Here's how the part is built. I have some questions about the finished solid (model axes, mm). A direction names the side the tool comes from. Give positions to 0.01 mm unless a question says otherwise; leave off trailing zeros. Loops run counter-clockwise (first coordinate to the right, second up) from the corner with the lowest first, then second, coordinate; pieces in that order, holes last. Notation, with made-up numbers: (45.5, 33.5) -> (49.5, 33.5) arc R27 ccw to (49.5, 52.5) -> close; hole circle Ø8 at (-22.75, 47.25). An arc over 180 degrees is marked (long way). Answer in a Markdown table with one row per item. Add a question column.
Item 1: If we section it at B-B (z = 14.5): Write out the boundary of the cut face in (x, y).
Item 2: If I drill on line 1 (Y direction, x = 10, z = 10); line 2 (Y direction, x = 18.85, z = 47); line 3 (Y direction, x = 7.25, z = 5.5), over which ranges is the centre line in solid material (lowest first)?
Item 3: Which directions (+Z, -Z, +X, -X, +Y, -Y) give clear straight access to the entire face, cutting with the end or side of a thin tool? Please do faces 1 (the face through (11.77, 16.62, -2.99)), 2 (the face through (10, 4.8, -2)), 3 (the face through (9, 32.3, 32)).
Item 4: We'd pull the mould along Z, two halves only. Please class faces 4 (the face through (9, 25, 61)), 5 (the face through (9, 9, 50.5)), 6 (the face through (10.14, 48.64, -2.43)), 7 (the face through (5.326, 36.472, -0.986)): released by +Z, released by -Z, zero draft, split by the parting line, or undercut.
Item 5: For P1, Ø1.2, axis at x = 13.5, z = -1.5, coming from the -Y side; P2, Ø1.2, axis at x = 8.5, y = 10.5, coming from the -Z side; P3, Ø1.5, axis at x = 10, y = 35.5, coming from the -Z side, each with a flat end and sliding along its axis, tell me the tip position at first contact or that it passes through.
Item 6: If we section it at A-A (z = 47): Write out the boundary of the cut face in (x, y).
Item 7: If we section it at D-D (z = 55): Write out the boundary of the cut face in (x, y), then the cut area to 3 significant figures.
Item 8: If we section it at C-C (y = 6): Write out the boundary of the cut face in (x, z).
```python
from build123d import *

# Parameters (mm, degrees)
SKETCH1_W           = 20
SKETCH1_H           = 50
BOSS_EXTRUDE1_DEPTH = 66
SKETCH2_R           = 4.9
BOSS_EXTRUDE2_DEPTH = 2
SKETCH3_R           = 2.4
BOSS_EXTRUDE3_DEPTH = 2
SKETCH4_R           = 1.5
CUT_EXTRUDE1_DEPTH  = 20
CUT_EXTRUDE2_START  = -18
CUT_EXTRUDE2_DEPTH  = 18
CUT_EXTRUDE3_REACH  = 86.735
SKETCH8_W           = 20
SKETCH8_H           = 4.8
BOSS_EXTRUDE4_DEPTH = 4
FILLET1_R           = 5


# Read off the part's stored shape, not the designer's step: Cut-Extrude2
with BuildPart() as part:
    # Sketch1 → Boss-Extrude1 (new body)
    with BuildSketch(Plane.XY):
        with Locations((10, 25)):
            Rectangle(SKETCH1_W, SKETCH1_H)
    extrude(amount=BOSS_EXTRUDE1_DEPTH)

    # Sketch2 → Boss-Extrude2 (add)
    with BuildSketch(Plane(origin=(0, 0, 0), x_dir=(-1, 0, 0), z_dir=(0, 0, -1))):
        with Locations((-10, 35)):
            Circle(SKETCH2_R)
        with Locations((-10, 15)):
            Circle(SKETCH2_R)
    extrude(amount=BOSS_EXTRUDE2_DEPTH)

    # Sketch3 → Boss-Extrude3 (add)
    with BuildSketch(Plane(origin=(0, 0, -2), x_dir=(-1, 0, 0), z_dir=(0, 0, -1))):
        with Locations((-10, 15)):
            Circle(SKETCH3_R)
        with Locations((-10, 35)):
            Circle(SKETCH3_R)
    extrude(amount=BOSS_EXTRUDE3_DEPTH)

    # Sketch4 → Cut-Extrude1 (cut)
    with BuildSketch(Plane(origin=(0, 0, -4), x_dir=(-1, 0, 0), z_dir=(0, 0, -1))):
        with Locations((-10, 15)):
            Circle(SKETCH4_R)
        with Locations((-10, 35)):
            Circle(SKETCH4_R)
    extrude(amount=-CUT_EXTRUDE1_DEPTH, mode=Mode.SUBTRACT)

    # Cut-Extrude2 outline → Cut-Extrude2 (cut)
    with BuildSketch(Plane.ZY.offset(CUT_EXTRUDE2_START)):
        with BuildLine():
            ThreePointArc((43.5, 38.555441712), (40.117469968, 37.191422409), (37.202041029, 35))
            Line((37.202041029, 35), (35.819660113, 35))
            ThreePointArc((35.819660113, 35), (34.783103517, 33.703300542), (33.896183762, 32.3))
            Line((33.896183762, 32.3), (31, 32.3))
            ThreePointArc((31, 32.3), (30.292893219, 32.007106781), (30, 31.3))
            Line((30, 31.3), (5, 31.3))
            Line((5, 31.3), (5, 18.7))
            Line((5, 18.7), (30, 18.7))
            ThreePointArc((30, 18.7), (30.292893219, 17.992893219), (31, 17.7))
            Line((31, 17.7), (33.896183762, 17.7))
            ThreePointArc((33.896183762, 17.7), (34.783103517, 16.296699458), (35.819660113, 15))
            Line((35.819660113, 15), (37.202041029, 15))
            ThreePointArc((37.202041029, 15), (40.117469968, 12.808577591), (43.5, 11.444558288))
            Line((43.5, 11.444558288), (43.5, 7.5))
            ThreePointArc((43.5, 7.5), (47, 4), (50.5, 7.5))
            Line((50.5, 7.5), (50.5, 11.444558288))
            ThreePointArc((50.5, 11.444558288), (61, 25), (50.5, 38.555441712))
            Line((50.5, 38.555441712), (50.5, 42.5))
            ThreePointArc((50.5, 42.5), (47, 46), (43.5, 42.5))
            Line((43.5, 42.5), (43.5, 38.555441712))
        make_face()
    extrude(amount=CUT_EXTRUDE2_DEPTH, mode=Mode.SUBTRACT)

    # Sketch7 → Cut-Extrude3 (cut, up to next)
    with BuildSketch(Plane.ZY.offset(-18), mode=Mode.PRIVATE) as cut_extrude3_sk1:
        with BuildLine():
            ThreePointArc((47, 40.25), (49.25, 42.5), (47, 44.75))
            ThreePointArc((47, 44.75), (44.75, 42.5), (47, 40.25))
        make_face()
    cut_extrude3_tool1 = extrude(cut_extrude3_sk1.sketch, amount=-CUT_EXTRUDE3_REACH, mode=Mode.PRIVATE) & part.part
    # Sketch7 → Cut-Extrude3 (cut, up to next)
    with BuildSketch(Plane.ZY.offset(-18), mode=Mode.PRIVATE) as cut_extrude3_sk2:
        with BuildLine():
            ThreePointArc((55, 20.5), (59.5, 25), (55, 29.5))
            ThreePointArc((55, 29.5), (50.5, 25), (55, 20.5))
        make_face()
    cut_extrude3_tool2 = extrude(cut_extrude3_sk2.sketch, amount=-CUT_EXTRUDE3_REACH, mode=Mode.PRIVATE) & part.part
    # Sketch7 → Cut-Extrude3 (cut, up to next)
    with BuildSketch(Plane.ZY.offset(-18), mode=Mode.PRIVATE) as cut_extrude3_sk3:
        with BuildLine():
            ThreePointArc((47, 5.25), (49.25, 7.5), (47, 9.75))
            ThreePointArc((47, 9.75), (44.75, 7.5), (47, 5.25))
        make_face()
    cut_extrude3_tool3 = extrude(cut_extrude3_sk3.sketch, amount=-CUT_EXTRUDE3_REACH, mode=Mode.PRIVATE) & part.part
    add(cut_extrude3_tool1.solids().sort_by_distance((18, 42.5, 47))[0], mode=Mode.SUBTRACT)
    add(cut_extrude3_tool2.solids().sort_by_distance((18, 25, 55))[0], mode=Mode.SUBTRACT)
    add(cut_extrude3_tool3.solids().sort_by_distance((18, 7.5, 47))[0], mode=Mode.SUBTRACT)

    # Sketch8 → Boss-Extrude4 (add)
    with BuildSketch(Plane(origin=(0, 0, 0), x_dir=(-1, 0, 0), z_dir=(0, 0, -1))):
        with Locations((-10, 2.4)):
            Rectangle(SKETCH8_W, SKETCH8_H)
        with Locations((-10, 47.6)):
            Rectangle(SKETCH8_W, SKETCH8_H)
    extrude(amount=BOSS_EXTRUDE4_DEPTH)

    # Fillet1
    # the kernel refuses this fillet: 5 mm, written as the material it takes off along each edge
    with BuildSketch(Plane(origin=(32.489995997, 0, -4), x_dir=(0, 0, 1), z_dir=(-1, 0, 0))) as fillet1_piece_1:
        with BuildLine():
            CenterArc((4.995998399, 5), FILLET1_R, 182.292442776, 87.707557224)
            Line((0, 4.8), (-0.099919968, 4.796))
            ThreePointArc((-0.099919968, 4.796), (-0.1, 2.4), (-0.1, 0))
            Line((-0.1, 0), (0, -0.1))
            Line((0, -0.1), (4.995998399, -0.1))
            Line((4.995998399, -0.1), (4.995998399, 0))
        make_face()
    extrude(amount=44.979991994, mode=Mode.SUBTRACT)
    with BuildSketch(Plane(origin=(32.489995997, 50, -4), x_dir=(0, -1, 0), z_dir=(-1, 0, 0))) as fillet1_piece_2:
        with BuildLine():
            CenterArc((5, 4.995998399), FILLET1_R, 180, 87.707557224)
            Line((0, 4.995998399), (-0.1, 4.995998399))
            Line((-0.1, 4.995998399), (-0.1, 0))
            Line((-0.1, 0), (0, -0.1))
            ThreePointArc((0, -0.1), (2.4, -0.1), (4.796, -0.099919968))
            Line((4.796, -0.099919968), (4.8, 0))
        make_face()
    extrude(amount=44.979991994, mode=Mode.SUBTRACT)
    with BuildSketch(Plane(origin=(32.5, 50, 66), x_dir=(0, 0, -1), z_dir=(-1, 0, 0)), Plane(origin=(-12.5, 0, 66), x_dir=(0, 0, -1), z_dir=(1, 0, 0))) as fillet1_piece_3:
        with BuildLine():
            CenterArc((FILLET1_R, FILLET1_R), FILLET1_R, 180, 90)
            Line((0, FILLET1_R), (-FILLET1_R * 0.02, FILLET1_R))
            Line((-FILLET1_R * 0.02, FILLET1_R), (-FILLET1_R * 0.02, -FILLET1_R * 0.02))
            Line((-FILLET1_R * 0.02, -FILLET1_R * 0.02), (FILLET1_R, -FILLET1_R * 0.02))
            Line((FILLET1_R, -FILLET1_R * 0.02), (FILLET1_R, 0))
        make_face()
    extrude(amount=45, mode=Mode.SUBTRACT)


solid = part.part
```
Recorded:
| question | item | result |
|---|---|---|
| 1 | outline | (0, 0) -> (20, 0) -> (20, 50) -> (0, 50) -> (0, 31.3) -> (18, 31.3) -> (18, 18.7) -> (0, 18.7) -> close; hole circle Ø3 at (10, 15); hole circle Ø3 at (10, 35) |
| 2 | line 1 | y = 0 to 13.5, 16.5 to 18.7, 31.3 to 33.5, 36.5 to 50 |
| 2 | line 2 | y = 0 to 5.25, 9.75 to 40.25, 44.75 to 50 |
| 2 | line 3 | y = 0 to 18.7, 31.3 to 50 |
| 3 | face 1 | -Z |
| 3 | face 2 | -Z, +X, -X |
| 3 | face 3 | -X |
| 4 | face 4 | undercut |
| 4 | face 5 | undercut |
| 4 | face 6 | released by -Z |
| 4 | face 7 | zero draft |
| 5 | P1 | stops at y = 0.37 |
| 5 | P2 | stops at z = -2 |
| 5 | P3 | stops at z = 16 |
| 6 | outline | (0, 0) -> (20, 0) -> (20, 5.25) -> (18, 5.25) -> (18, 4) -> (0, 4) -> close; (0, 46) -> (18, 46) -> (18, 44.75) -> (20, 44.75) -> (20, 50) -> (0, 50) -> close; (18, 9.75) -> (20, 9.75) -> (20, 40.25) -> (18, 40.25) -> close |
| 7 | outline | (0, 0) -> (20, 0) -> (20, 20.5) -> (18, 20.5) -> (18, 13.51) -> (0, 13.51) -> close; (0, 36.49) -> (18, 36.49) -> (18, 29.5) -> (20, 29.5) -> (20, 50) -> (0, 50) -> close |
| 7 | area | 568 mm^2 |
| 8 | outline | (0, 0) -> (20, 0) -> (20, 45.32) -> (18, 45.32) -> (18, 43.84) -> (0, 43.84) -> close; (0, 50.16) -> (18, 50.16) -> (18, 48.68) -> (20, 48.68) -> (20, 66) -> (0, 66) -> close |
